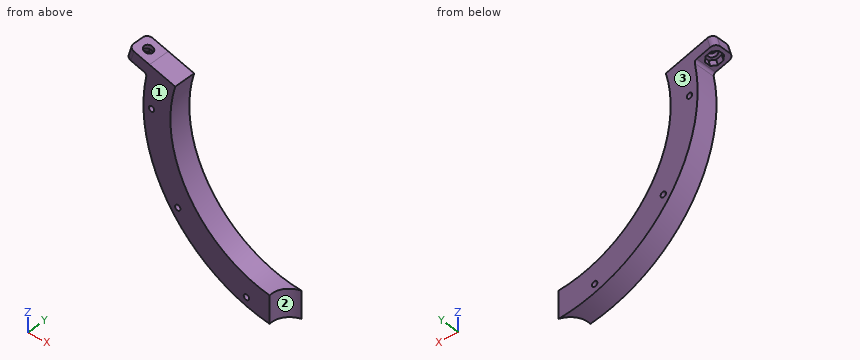
Autodesk Inventor part; units mm, degrees
ref_plane "YZ Plane" through (0, 0, 0) normal (1, 0, 0) x (0, 1, 0)
ref_plane "XZ Plane" through (0, 0, 0) normal (0, 1, 0) x (-1, 0, 0)
ref_plane "XY Plane" through (0, 0, 0) normal (0, 0, 1) x (1, 0, 0)
sketch "Sketch1" plane through (0, 0, 0) normal (0, 1, 0) x (-1, 0, 0)
  circle A0 centre (0, 0) radius 135
  circle A1 centre (0, 0) radius 110
  dimension "d0" = 270
  dimension "d1" = 220
extrude "Extrusion1" add sketch "Sketch1" along normal mid plane 47
sketch "Sketch2" plane through (0, 0, 0) normal (0, 0, 1) x (1, 0, 0)
  circle A0 centre (0, -20.5) radius 18
  line L0 (-135, -23.5) -> (135, -23.5)
  dimension "d4" = 36
  dimension "d38" = 3
extrude "Extrusion2" cut sketch "Sketch2" against normal through all
sketch "Sketch3" plane through (0, 23.5, 0) normal (0, 1, 0) x (1, 0, 0)
  circle A0 centre (0, 0) radius 127.5
  circle A1 centre (-127.5, 0) radius 2
  circle A2 centre (-103.1497, -74.9426) radius 2
  circle A3 centre (-39.3997, -121.2597) radius 2
  circle A4 centre (39.3997, -121.2597) radius 2
  circle A5 centre (103.1497, -74.9426) radius 2
  circle A6 centre (127.5, 0) radius 2
  circle A7 centre (103.1497, 74.9426) radius 2
  circle A8 centre (39.3997, 121.2597) radius 2
  circle A9 centre (-39.3997, 121.2597) radius 2
  circle A10 centre (-103.1497, 74.9426) radius 2
  dimension "d7" = 255
  dimension "d8" = 4
  dimension "d11" = 360
hole "Hole1" at (39.3997, 23.5, 121.2597) at (-39.3997, 23.5, 121.2597) at (-103.1497, 23.5, 74.9426) at (-127.5, 23.5, 0) at (-103.1497, 23.5, -74.9426) at (-39.3997, 23.5, -121.2597) at (39.3997, 23.5, -121.2597) at (103.1497, 23.5, -74.9426) at (127.5, 23.5, 0) at (103.1497, 23.5, 74.9426) direction (0, -1, 0) diameter 5 end through all
sketch "Sketch4" plane through (0, 23.5, 0) normal (0, 1, 0) x (1, 0, 0)
  circle A0 centre (0, 0) radius 140
extrude "Extrusion3" cut sketch "Sketch4" against normal blind 27
sketch "Sketch7" plane through (0, -3.5, 0) normal (0, 1, 0) x (1, 0, 0)
  line L0 (0, 0) -> (70, 0)
  line L1 (80, -100) -> (60, -100)
  line L2 (60, -100) -> (60, 100)
  line L3 (60, 100) -> (80, 100)
  line L4 (80, 100) -> (80, -100)
  line L5 (80, -100) -> (60, 100) construction
  line L6 (60, -100) -> (80, 100) construction
  dimension "d39" = 70
  dimension "d40" = 20
  dimension "d41" = 200
extrude "Extrusion7" cut sketch "Sketch7" against normal blind 15
sketch "Sketch8" plane through (0, -3.5, 0) normal (0, 1, 0) x (1, 0, 0)
  line L0 (-129.4827, -38.1999) -> (129.4827, 38.1999)
  line L1 (0, 134.8703) -> (0, -135)
  arc A0 (-5.9161, 134.8703) -> (5.9161, 134.8703) centre (0, 0) ccw
  arc A1 (129.4827, 38.1999) -> (0, 135) centre (0, 0) ccw
extrude "Extrusion8" cut sketch "Sketch8" against normal through all
sketch "Sketch9" plane through (0, -3.5, 0) normal (0, 1, 0) x (1, 0, 0)
  line L0 (129.4827, 38.1999) -> (105.5044, 31.1258)
  arc A0 (105.5044, 31.1258) -> (17.7482, 108.5587) centre (0, 0) ccw
  line L1 (17.7482, 108.5587) -> (17.7482, 133.8282)
  arc A1 (129.4827, 38.1999) -> (17.7482, 133.8282) centre (0, 0) ccw
  circle A2 centre (39.3997, 121.2597) radius 2.5
  circle A3 centre (103.1497, 74.9426) radius 2.5
  line L2 (105.5044, 31.1258) -> (129.4827, 38.1999)
  arc A4 (129.4827, 38.1999) -> (5.9161, 134.8703) centre (0, 0) ccw
  line L3 (5.9161, 109.8408) -> (5.9161, 134.8703)
  arc A5 (60, 92.1954) -> (5.9161, 109.8408) centre (0, 0) ccw
  line L4 (60, 92.1954) -> (60, 100)
  line L5 (60, 100) -> (80, 100)
  line L6 (80, 100) -> (80, 75.4983)
  arc A6 (105.5044, 31.1258) -> (80, 75.4983) centre (0, 0) ccw
  circle A7 centre (103.1497, 74.9426) radius 2.5
  circle A8 centre (39.3997, 121.2597) radius 2.5
  point P0 (17.7482, 108.5587)
extrude "Extrusion9" cut sketch "Sketch9" against normal through all
sketch "Sketch10" plane through (-105.5044, -23.5, 31.1258) normal (0.2829619, 0, 0.9591312) x (0.9591312, 0, -0.2829619)
  line L0 (-25, 0) -> (130.8454, 0)
  line L1 (-22.5, 0) -> (-40, 0)
  line L2 (-45, 5) -> (-45, 15)
  line L3 (-40, 20) -> (-22.5, 20)
  line L4 (-22.5, 20) -> (-22.5, 0)
  line L5 (-25, 0) -> (-25, 20)
  arc A0 (-45, 5) -> (-40, 0) centre (-40, 5) ccw
  arc A1 (-40, 20) -> (-45, 15) centre (-40, 15) ccw
  point P0 (110, 23.5)
  point P1 (-45, 20)
  point P2 (-45, 0)
  point P3 (-25, 0)
  dimension "d48" = 22.5
  dimension "d49" = 20
  dimension "d50" = 20
  dimension "d51" = 5
extrude "Extrusion10" add sketch "Sketch10" against normal blind 10
fillet "Fillet1" radius 2.5 1 edges at (-131.9566, -13.5, 28.5036)
sketch "Sketch11" plane through (-108.334, -23.5, 21.5345) normal (-0.2829619, 0, -0.9591312) x (-0.9591312, 0, 0.2829619)
  line L0 (32.2662, 16.6) -> (37.7338, 16.6)
  line L1 (37.7338, 16.6) -> (41.6, 12.7338)
  line L2 (41.6, 12.7338) -> (41.6, 7.2662)
  line L3 (41.6, 7.2662) -> (37.7338, 3.4)
  line L4 (37.7338, 3.4) -> (32.2662, 3.4)
  line L5 (32.2662, 3.4) -> (28.4, 7.2662)
  line L6 (28.4, 7.2662) -> (28.4, 12.7338)
  line L7 (28.4, 12.7338) -> (32.2662, 16.6)
  line L8 (40, 20) -> (26.9306, 20)
  line L9 (45, 5) -> (45, 15)
  point P0 (-110, 23.5)
  point P1 (35, 10)
  dimension "d55" = 10
  dimension "d56" = 10
  dimension "d57" = 13.2
extrude "Extrusion11" cut sketch "Sketch11" against normal blind 6
sketch "Sketch12" plane through (-106.6363, -23.5, 27.2893) normal (-0.2829619, 0, -0.9591312) x (-0.9591312, 0, 0.2829619)
  line L0 (45, 5) -> (45, 15)
  line L1 (40, 20) -> (26.9306, 20)
  point P0 (-110, 23.5)
  point P1 (35, 10)
  dimension "d60" = 10
  dimension "d61" = 10
hole "Hole2" at (-140.2059, -13.5, 37.1929) direction (0.2829619, 0, 0.9591312) diameter 8.2 end through all
properties part number "Cylinder Spacer Bottom_Q"
Read the model definition and answer for the solid it produces. Units are mm, in the model's axes. Face numbers are marked on the shaded views. Round coordinates to 2 decimals unless told otherwise and drop trailing zeros. Write each loop counter-clockwise with the first axis right and the second up, starting at its lowest first coordinate (ties: lowest second). Pieces come first, ordered by that corner, then holes.
1. Given pin 1 Ø2 at (x, y) = (-109.5, -12.5) entering from -Z; pin 2 Ø4.5 at (x, z) = (-127.5, 0) entering from -Y; pin 3 Ø12 at (x, y) = (-28, -18) entering from +Z; pin 4 Ø5 at (x, y) = (-50, -14) entering from -Z, each flat-ended and moving along its own axis, determine where each tip first touches the part or whether it passes through.
2. The part is cut by section D-D, the plane z = -115.5. Determine the outline of the cut face in (x, y), then the cut area to 3 significant figures.
3. Straight lines are drawn through the part: L1, parallel to X at y = -19.25, z = -119; L2, parallel to Y at x = -135, z = 35.5; L3, parallel to X at y = -19, z = -36.5. For each, find the intervals that lie inside material, in ascending order.
4. The part is cut by section A-A, the plane z = 0. Determine the outline of the cut face in (x, y), then the cut area to 3 significant figures.
5. The part is cut by section B-B, the plane x = -127.5. Determine the outline of the cut face in (y, z), then the cut area to 3 significant figures.
6. Determine the mould class of the marked faces 1, 2 and 3 for opening direction Y: pulls with the +Y half, pulls with the -Y half, needs draft (parallel to the pull), parting line crosses it, or undercut.
7. The part is cut by section C-C, the plane x = -49. Determine the outline of the cut face in (y, z), then the cut area to 3 significant figures.
Values:
1. pin 1: stops at z = -80.33
1. pin 2: passes through
1. pin 3: stops at z = -104.61
1. pin 4: stops at z = -126.37
2. outline: (-69.89, -23.5) - (-17.75, -23.5) arc R18 cw to (-5.92, -3.5) - (-69.89, -3.5) - close
2. area: 1,090 mm2
3. L1: x = -63.75 to -40.47, -38.33 to -17.96
3. L2: y = -23.5 to -17.36, -9.64 to -3.5
3. L3: x = -129.97 to -103.77
4. outline: (-135, -23.5) - (-130, -23.5) - (-130, -3.5) - (-135, -3.5) - close; (-125, -23.5) - (-110, -23.5) - (-110, -3.5) - (-125, -3.5) - close
4. area: 400 mm2
5. outline: (-23.5, -44.37) - (-3.5, -44.37) - (-3.5, -2.5) - (-23.5, -2.5) - close; (-23.5, 2.5) - (-3.5, 2.5) - (-3.5, 37.61) - (-23.5, 37.61) - close
5. area: 1,540 mm2
6. face 1: pulls with the -Y half
6. face 2: undercut
6. face 3: pulls with the +Y half
7. outline: (-23.5, -125.79) - (-3.5, -125.79) - (-3.5, -98.48) - (-23.5, -98.48) - close
7. area: 546 mm2
